Geometry check sheet. Reference: the model listing, model coordinates, mm. Face numbers are marked on the shaded views. A direction names the side the tool comes from. Give positions to 0.01 mm unless a question says otherwise; leave off trailing zeros. Order: outer loops, then holes, each group sorted by start corner. A loop starts at its lowest first (then second) coordinate and runs counter-clockwise, first axis right, second up.
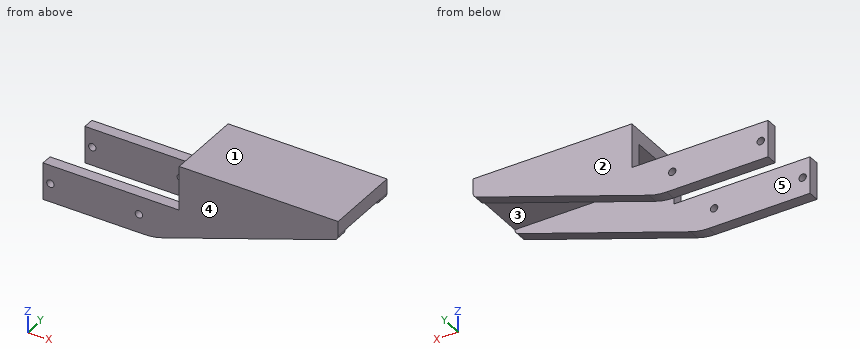
```python
from build123d import *

# Parameters (mm, degrees)
BOSS_EXTRUDE1_DEPTH                      = 3
BOSS_EXTRUDE2_START                      = 15
BOSS_EXTRUDE2_DEPTH                      = 3
SKETCH3_W                                = 1
SKETCH3_H                                = 21
F_2_0MM_CLEARANCE_DOWEL_HOLE1_AT_2_COUNT = 2
F_2_0MM_CLEARANCE_DOWEL_HOLE1_AT_2_PITCH = 24
SKETCH5_W                                = 43.073811931
SKETCH5_H                                = 3.925670489
BOSS_EXTRUDE3_DEPTH                      = 15


with BuildPart() as part:
    # Sketch1 → Boss-Extrude1 (new body)
    with BuildSketch(Plane(origin=(0, 0, 0), x_dir=(1, 0, 0), z_dir=(0, 1, 0))):
        with BuildLine():
            Line((-4.577926811, 9.356292891), (42.056666031, -6.499468675))
            ThreePointArc((42.056666031, -6.499468675), (42.793295664, -7.04620955), (43.073811931, -7.919627792))
            Line((43.073811931, -7.919627792), (43.073811931, -11.845298281))
            Line((43.073811931, -11.845298281), (0, -11.845298281))
            Line((0, -11.845298281), (0, 0.154701719))
            Line((0, 0.154701719), (-36.926188069, 0.154701719))
            Line((-36.926188069, 0.154701719), (-36.926188069, 10.154701719))
            Line((-36.926188069, 10.154701719), (-9.406467809, 10.154701719))
            ThreePointArc((-9.406467809, 10.154701719), (-6.959415254, 9.953753506), (-4.577926811, 9.356292891))
        make_face()
    extrude(amount=-BOSS_EXTRUDE1_DEPTH)


with BuildPart() as body_2:
    # Sketch1<2> → Boss-Extrude2 (new body)
    with BuildSketch(Plane(origin=(0, 0, 0), x_dir=(1, 0, 0), z_dir=(0, 1, 0)).offset(BOSS_EXTRUDE2_START)):
        with BuildLine():
            Line((-4.577926811, 9.356292891), (42.056666031, -6.499468675))
            ThreePointArc((42.056666031, -6.499468675), (42.793295664, -7.04620955), (43.073811931, -7.919627792))
            Line((43.073811931, -7.919627792), (43.073811931, -11.845298281))
            Line((43.073811931, -11.845298281), (0, -11.845298281))
            Line((0, -11.845298281), (0, 0.154701719))
            Line((0, 0.154701719), (-36.926188069, 0.154701719))
            Line((-36.926188069, 0.154701719), (-36.926188069, 10.154701719))
            Line((-36.926188069, 10.154701719), (-9.406467809, 10.154701719))
            ThreePointArc((-9.406467809, 10.154701719), (-6.959415254, 9.953753506), (-4.577926811, 9.356292891))
        make_face()
    extrude(amount=BOSS_EXTRUDE2_DEPTH)


with BuildPart() as f_2_0mm_clearance_dowel_hole1_tool:
    # Sketch3 → Ø2.0mm Clearance Dowel Hole1 (revolve)
    with BuildSketch(Plane(origin=(-34.926188069, -3, -5.154701719), x_dir=(0, 0, -1), z_dir=(1, 0, 0))):
        with Locations((0.5, 10.5)):
            Rectangle(SKETCH3_W, SKETCH3_H)
    f_2_0mm_clearance_dowel_hole1 = revolve(axis=Axis((-34.926188069, -9.35, -5.154701719), (0, 1, 0)))


with BuildPart() as part_1:
    add(part.part)

    # Ø2.0mm Clearance Dowel Hole1: cut by f_2_0mm_clearance_dowel_hole1_tool
    add(f_2_0mm_clearance_dowel_hole1_tool.part, mode=Mode.SUBTRACT)


with BuildPart() as body_2_1:
    add(body_2.part)

    # Ø2.0mm Clearance Dowel Hole1: cut by f_2_0mm_clearance_dowel_hole1_tool
    add(f_2_0mm_clearance_dowel_hole1_tool.part, mode=Mode.SUBTRACT)


with BuildPart() as f_2_0mm_clearance_dowel_hole1_at_2_tool:
    # Ø2.0mm Clearance Dowel Hole1 at 2: Ø2.0mm Clearance Dowel Hole1 ×2
    with Locations(*[(i * F_2_0MM_CLEARANCE_DOWEL_HOLE1_AT_2_PITCH, 0, 0) for i in range(1, F_2_0MM_CLEARANCE_DOWEL_HOLE1_AT_2_COUNT)]):
        add(f_2_0mm_clearance_dowel_hole1)


with BuildPart() as part_2:
    add(part_1.part)

    # Ø2.0mm Clearance Dowel Hole1 at 2: cut by f_2_0mm_clearance_dowel_hole1_at_2_tool
    add(f_2_0mm_clearance_dowel_hole1_at_2_tool.part, mode=Mode.SUBTRACT)



with BuildPart() as body_2_2:
    add(body_2_1.part)

    # Ø2.0mm Clearance Dowel Hole1 at 2: cut by f_2_0mm_clearance_dowel_hole1_at_2_tool
    add(f_2_0mm_clearance_dowel_hole1_at_2_tool.part, mode=Mode.SUBTRACT)


with BuildPart() as part_3:
    add(part_2.part)

    add(body_2_2.part)  # Boss-Extrude3 merges body 2
    # Sketch5 → Boss-Extrude3 (add)
    with BuildSketch(Plane(origin=(0, 0, 0), x_dir=(1, 0, 0), z_dir=(0, 1, 0))):
        with Locations((21.536905966, -9.882463037)):
            Rectangle(SKETCH5_W, SKETCH5_H)
    extrude(amount=BOSS_EXTRUDE3_DEPTH)


solid = part_3.part
```
Q1. Cross-section at D-D, the plane y = 13.25. Record the boundary of the cut face in (x, z).
Q2. Gauge pin test, flat ends, axial feed: P1, Ø12, axis at x = 22.5, y = 6.5, coming from the -Z side; P2, Ø1.2, axis at x = -34.93, z = -5.15, coming from the -Y side; P3, Ø8, axis at y = 1, z = 6.5, coming from the -X side; P4, Ø1.5, axis at x = -23, y = -1.5, coming from the +Z side. Record the tip position at first contact, or that the pin passes through.
Q3. Access from +Z, -Z, +X, -X, +Y, -Y to the whole of each face (thin tool, end or side, straight path). Record for the marked faces 4 and 5.
Q4. Cross-section at C-C, the plane x = 15. Record the boundary of the cut face in (y, z).
Q5. Thickness scan on L1, parallel to Y at x = -32.5, z = -6.25; L2, parallel to X at y = 15.5, z = 8.75; L3, parallel to Z at x = 4.5, y = 2. Record the ranges inside material, lowest first.
Q6. Cross-section at B-B, the plane z = -8. Record the boundary of the cut face in (x, y).
Q7. Release check for a two-part mould opening along Y. For the marked faces 1, 2 and 3 record: pulls with the +Y half, pulls with the -Y half, needs draft (parallel to the pull), parting line crosses it, or undercut.
Q8. Cross-section at A-A, the plane x = -29. Record the boundary of the cut face in (y, z).
Answers follow:
1. outline: (0, 7.92) - (43.07, 7.92) - (43.07, 11.85) - (0, 11.85) - close
2. P1: stops at z = 7.92
2. P2: passes through
2. P3: stops at x = 0
2. P4: stops at z = -0.15
3. face 4: +Z, -Z, +X, -X, -Y
3. face 5: -Z, +X, -X
4. outline: (-3, -2.7) - (0, -2.7) - (0, 7.92) - (15, 7.92) - (15, -2.7) - (18, -2.7) - (18, 11.85) - (-3, 11.85) - close
5. L1: y = -3 to 0, 15 to 18
5. L2: x = 0 to 43.07
5. L3: z = 7.92 to 11.85
6. outline: (-36.93, -3) - (-0.59, -3) - (-0.59, 0) - (-36.93, 0) - close; (-36.93, 15) - (-0.59, 15) - (-0.59, 18) - (-36.93, 18) - close
7. face 1: needs draft
7. face 2: pulls with the +Y half
7. face 3: undercut
8. outline: (-3, -10.15) - (0, -10.15) - (0, -0.15) - (-3, -0.15) - close; (15, -10.15) - (18, -10.15) - (18, -0.15) - (15, -0.15) - close
